Here's how the part is built. I have some questions about the finished solid (model axes, mm). Round coordinates to 2 decimals unless told otherwise and drop trailing zeros. Loops run counter-clockwise (first coordinate to the right, second up) from the corner with the lowest first, then second, coordinate; pieces in that order, holes last. Notation, with made-up numbers: M 9.5,-1 L 65.5,-1 A16 cw 65.5,26 Z; hole C 52,39 d9. An arc over 180 degrees is marked long. Write item = value, one per line. Start each with the question number.
from build123d import *

# Parameters (mm, degrees)
SKETCH_1_R          = 9.5
SKETCH_1_R_2        = 5
SKETCH_1_R_3        = 4
EXTRUDE_2_DEPTH     = 6
SKETCH_2_W          = 12
SKETCH_2_H          = 28
CUT_EXTRUDE_1_DEPTH = 6
EXTRUDE_START       = -1
SKETCH_4_R          = 9.5
SKETCH_4_R_2        = 8
EXTRUDE_4_DEPTH     = 1


with BuildPart() as part:
    # 草图1 → 凸台-拉伸2 (new body)
    with BuildSketch(Plane.XY):
        with BuildLine():
            Line((-8, -127.68857754), (-8, -107.68857754))
            ThreePointArc((-8, -107.68857754), (-13.133925537, -102.245688373), (-15, -95))
            Line((-15, -95), (-15, 95))
            ThreePointArc((-15, 95), (0, 110), (15, 95))
            Line((15, 95), (15, -95))
            ThreePointArc((15, -95), (13.133925537, -102.245688373), (8, -107.68857754))
            Line((8, -107.68857754), (8, -127.68857754))
            ThreePointArc((8, -127.68857754), (0, -135.68857754), (-8, -127.68857754))
        make_face()
        with Locations((0, 95)):
            Circle(SKETCH_1_R, mode=Mode.SUBTRACT)
        with Locations((0, -95)):
            Circle(SKETCH_1_R_2, mode=Mode.SUBTRACT)
        with Locations((0, -127.68857754)):
            Circle(SKETCH_1_R_3, mode=Mode.SUBTRACT)
    extrude(amount=EXTRUDE_2_DEPTH)

    # 草图2 → 切除-拉伸1 (cut)
    with BuildSketch(Plane.XY.offset(6)):
        with Locations((0, 60)):
            Rectangle(SKETCH_2_W, SKETCH_2_H)
        with Locations((0, 20)):
            Rectangle(SKETCH_2_W, SKETCH_2_H)
        with Locations((0, -20)):
            Rectangle(SKETCH_2_W, SKETCH_2_H)
        with Locations((0, -60)):
            Rectangle(SKETCH_2_W, SKETCH_2_H)
    extrude(amount=-CUT_EXTRUDE_1_DEPTH, mode=Mode.SUBTRACT)

    # 草图4 → 凸台-拉伸4 (add)
    with BuildSketch(Plane.XY.offset(6).offset(EXTRUDE_START)):
        with Locations((0, 95)):
            Circle(SKETCH_4_R)
        with Locations((0, 95)):
            Circle(SKETCH_4_R_2, mode=Mode.SUBTRACT)
    extrude(amount=EXTRUDE_4_DEPTH)


solid = part.part
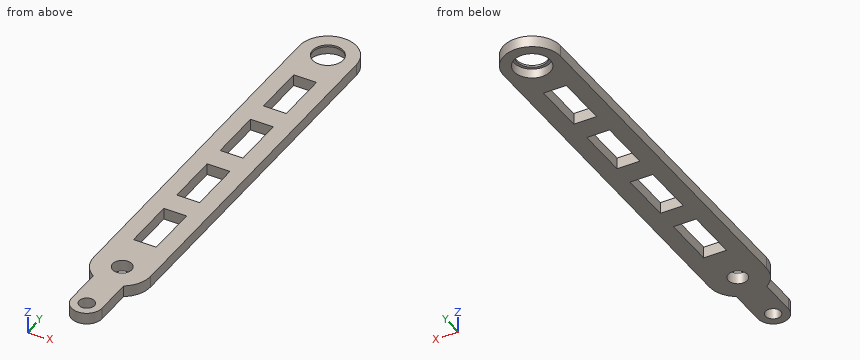
Item 1: Please list where these lines run through material, in increasing order: line 1 (X direction, y = -57.5, z = 2.85); line 2 (Y direction, x = 5.5, z = 2.6); line 3 (Y direction, x = -8.5, z = 0.5). Write a range as [from, to].
Item 2: Will these pins go through, and if not, where does the flat tip stop? pin 1 Ø1.8 at (x, z) = (-3, 2) entering from +Y; pin 2 Ø3 at (x, z) = (-8.5, 3) entering from +Y.
Item 3: I want a section at D-D, the plane y = -104. List the corners of the cut face in (x, z) for me, then the cut area to 3 significant figures.
Item 4: I want a section at A-A, the plane y = -32. List the corners of the cut face in (x, z) for me.
Item 5: I want a section at C-C, the plane x = 0. State how many separate pieces and enclosed holes the cut face has, then the cut area to 3 significant figures.
Item 6: I want a section at B-B, the plane z = 1.4. List the corners of the cut face in (x, y) for me, then the cut area to 3 significant figures.
Worked out:
q1.line_1 = [-15, -6], [6, 15]
q1.line_2 = [-133.5, -74], [-46, -34], [-6, 6], [34, 46], [74, 87.25], [102.75, 108.96]
q1.line_3 = [-107.36, 90.76], [99.24, 107.36]
q2.pin_1 = 109.85
q2.pin_2 = 108.27
q3.outline = M -12,0 L 12,0 L 12,6 L -12,6 Z
q3.area = 144 mm2
q4.outline = M -15,0 L -6,0 L -6,6 L -15,6 Z; M 6,0 L 15,0 L 15,6 L 6,6 Z
q5.separate_pieces = 8
q5.enclosed_holes = 0
q5.area = 583 mm2
q6.outline = M -15,-95 A15 ccw -8,-107.69 L -8,-127.69 A8 ccw 8,-127.69 L 8,-107.69 A15 ccw 15,-95 L 15,95 A15 ccw -15,95 Z; hole C 0,95 d19; hole M -6,-74 L 6,-74 L 6,-46 L -6,-46 Z; hole M -6,-34 L 6,-34 L 6,-6 L -6,-6 Z; hole M -6,6 L 6,6 L 6,34 L -6,34 Z; hole M -6,46 L 6,46 L 6,74 L -6,74 Z; hole C 0,-95 d10; hole C 0,-127.69 d8
q6.area = 5,050 mm2
